```python
from build123d import *

# Parameters (mm, degrees)
F0_R     = 31.75
F0_R_2   = 8.3458742529
F1_DEPTH = 38.1
F2_T     = -2.54
F3_R     = 19.05
F3_R_2   = 8.3458742529
F4_DEPTH = 25.4
F6_T     = -2.54


# Not quite as in the source:
# - a fillet or chamfer that OpenCascade refuses, or shapes differently, is made with other operations: its cross-section is extruded or revolved along the edge and cut away or added
# - the program builds the solid bodies; features that only make, move or delete a surface that nothing else refers to are left out


with BuildPart() as f1:
    # F0 (on Top) → F1 (new body)
    with BuildSketch(Plane.XY):
        Circle(F0_R)
        Circle(F0_R_2, mode=Mode.SUBTRACT)
    extrude(amount=F1_DEPTH)

    # F2
    f2_openings = [f1.faces().sort_by_distance(p)[0] for p in [
        (-30.851974, 0, 0),
        (-8.345874, 0, 19.05),
    ]]
    offset(amount=F2_T, openings=f2_openings)

    # F3 (on face) → F4 (join)
    with BuildSketch(Plane.XY.offset(38.1)):
        Circle(F3_R)
        Circle(F3_R_2, mode=Mode.SUBTRACT)
    extrude(amount=F4_DEPTH)

    # F6
    f6_openings = [f1.faces().sort_by_distance(p)[0] for p in [
        (-18.511185, 0, 63.5),
        (-8.345874, 0, 49.53),
    ]]
    offset(amount=F6_T, openings=f6_openings, kind=Kind.INTERSECTION)

    # F7: chamfer of 5.08 on 1 edges, made by hand

    # F7_s1 → F7_t2 (revolve, cut)
    with BuildSketch(Plane.XZ):
        Polygon((34.29, 0), (29.21, 5.08), (29.21, 0), align=None)
    revolve(axis=Axis((0, 0, 0), (0, 0, 1)), mode=Mode.SUBTRACT)


solid = f1.part
```
The listing builds one solid part. Answer for the finished solid, in the listing's coordinates (mm). A direction names the side the tool comes from. Coordinates: 2 decimals unless noted, no trailing zeros. Loops run counter-clockwise (first coordinate to the right, second up) from the corner with the lowest first, then second, coordinate; pieces in that order, holes last. Notation, with made-up numbers: M 39,-25 L 88,-25 A12 ccw 88,-16 Z; hole C 51,-21 d6. An arc over 180 degrees is marked long. Answer as CSV lines item,"result". Start each with the question number.
(1) For faces 1 (the flat face through (6.1, -6.1, 35.56)), 2 (the cylindrical face through (7.96, 2.51, 36.81)), 3 (the cylindrical face through (15.748, 4.959, 50.622)), determine the directions among +Z, -Z, +X, -X, +Y, -Y from which every point of the face is accessible in a straight line to the end or side of a thin tool.
(2) Given pin 1 (8 mm diameter, centred on x = 16, y = -0.5, fed in from -Z); pin 2 (10 mm diameter, centred on y = 5.5, z = 12.5, fed in from -X); pin 3 (10 mm diameter, centred on x = -7.5, y = -1.5, fed in from +Z), each flat-ended and moving along its own axis, determine where each tip first touches the part or whether it passes through.
(3) The mould has two halves that part along Y. Classify faces 4 (the cylindrical face through (-15.12, -11.59, 50.62)), 5 (the flat face through (14, -14, 38.1)), 6 (the cylindrical face through (-21.53, 19.74, 20.11)): pulls with the +Y half, pulls with the -Y half, needs draft (parallel to the pull), parting line crosses it, or undercut.
(4) The part is cut by section C-C (z = 40). Give the vertices of the cut face in (x, y), and give its area (3 significant figures).
(5) Find the intervals of material crossed by L1, parallel to X at y = -1, z = 9; L2, parallel to Y at x = -0.5, z = 46, in increasing order. Write a range as [from, to].
(6) The part is cut by section D-D (z = 10). Give the vertices of the cut face in (x, y), and give its area (3 significant figures).
(7) The part is cut by section A-A (y = 0). Give the vertices of the cut face in (x, z).
Determined:
1,face 1,"-Z"
1,face 2,"+Z, -Z"
1,face 3,"+Z"
2,pin 1,"z = 35.56"
2,pin 2,"x = -31.75"
2,pin 3,"z = 38.1"
3,face 4,"parting line crosses it"
3,face 5,"needs draft"
3,face 6,"undercut"
4,outline,"C 0,0 d38.1; hole C 0,0 d33.02"
4,area,"284 mm2"
5,L1,"[-31.73, -29.19], [29.19, 31.73]"
5,L2,"[-19.04, -16.5], [16.5, 19.04]"
6,outline,"C 0,0 d63.5; hole C 0,0 d58.42"
6,area,"486 mm2"
7,outline,"M -31.75,2.54 L -29.21,5.08 L -29.21,35.56 L -8.35,35.56 L -8.35,38.1 L -16.51,38.1 L -16.51,63.5 L -19.05,63.5 L -19.05,38.1 L -31.75,38.1 Z; M 8.35,35.56 L 29.21,35.56 L 29.21,5.08 L 31.75,2.54 L 31.75,38.1 L 19.05,38.1 L 19.05,63.5 L 16.51,63.5 L 16.51,38.1 L 8.35,38.1 Z"
